For this review, take the finished solid that the model builds, in its own axes (mm). A direction names the side the tool comes from. Round coordinates to 2 decimals unless told otherwise and drop trailing zeros. Order: outer loops, then holes, each group sorted by start corner. A loop starts at its lowest first (then second) coordinate and runs counter-clockwise, first axis right, second up. Notation, with made-up numbers: (-22, 5) -> (17, 5) arc R10 ccw to (17, 22) -> close; hole circle Ø10 at (60, 80.5). An arc over 180 degrees is marked (long way). Put each result on its own line as item: value. Start each with the question number.
```python
from build123d import *

# Parameters (mm, degrees)
F0_W     = 67.1
F0_H     = 138.3
F1_DEPTH = 3.55
F2_R     = 5
F3_T     = -2.5
F4_R     = 5
F6_DEPTH = 25


with BuildPart() as f1:
    # F0 (on Front) → F1 (new body, symmetric)
    with BuildSketch(Plane.XZ):
        with Locations((0, -4.651891)):
            Rectangle(F0_W, F0_H)
    extrude(amount=F1_DEPTH, both=True)

    # F2
    f2_edges = [f1.edges().sort_by_distance(p)[0] for p in [
        (-33.55, 0, 64.498109),
        (33.55, 0, 64.498109),
        (33.55, 0, -73.801891),
        (-33.55, 0, -73.801891),
    ]]
    fillet(f2_edges, radius=F2_R)

    # F3
    f3_openings = [f1.faces().sort_by_distance(p)[0] for p in [
        (0, -3.55, -4.651891),
    ]]
    offset(amount=F3_T, openings=f3_openings)

    # F4
    f4_edges = [f1.edges().sort_by_distance(p)[0] for p in [
        (33.55, 3.55, -4.651891),
        (32.085534, 3.55, -72.337424),
        (32.085534, 3.55, 63.033643),
        (0, 3.55, -73.801891),
        (0, 3.55, 64.498109),
        (-32.085534, 3.55, -72.337424),
        (-32.085534, 3.55, 63.033643),
        (-33.55, 3.55, -4.651891),
    ]]
    fillet(f4_edges, radius=F4_R)

    # F5 (on Front) → F6 (cut)
    with BuildSketch(Plane.XZ):
        with BuildLine():
            add(Edge.make_bspline(
                [(27.755955, 53.217217), (27.755955, 64.267715), (15.384319, 58.742466), (3.012683, 53.217217), (15.384319, 47.691968), (27.755955, 42.166719), (27.755955, 53.217217)],
                knots=[0, 0, 0, 2.094395, 2.094395, 4.18879, 4.18879, 6.283185, 6.283185, 6.283185], degree=2, weights=[1, 0.5, 1, 0.5, 1, 0.5, 1]))
        make_face()
    extrude(amount=-F6_DEPTH, mode=Mode.SUBTRACT)


solid = f1.part
```
Item 1: Mouldability with a two-part tool opening along Z and no side actions: class faces 3 (the face through (-32.12, -2.51, -72.3)), 4 (the face through (-32.124, -2.485, 62.995)), 5 (the face through (-30.337, -1.218, 61.246)) as +Z half, -Z half, draft (parallel to the pull), parting line (faces both ways), or undercut.
Item 2: Consider section B-B, the plane z = -2.5. Write out the cut boundary in (x, y), plus the area to 3 significant figures.
Item 3: Tool access review of faces 1 (the face through (31.05, -1, -6)), 2 (the face through (32.124, -2.485, 62.995)): name each direction out of +Z, -Z, +X, -X, +Y, -Y from which nothing blocks a thin tool from reaching the whole face with its end or side.
Item 4: For L1, parallel to Z at x = -11.5, y = -2; L2, parallel to X at y = -2.25, z = -56.5, list the stretches that pass through material, from the lowest coordinate up.
Item 5: Consider section A-A, the plane x = -11. Write out the cut boundary in (y, z), plus the area to 3 significant figures.
Item 6: Insertion check: pin 1 Ø2 at (x, y) = (0, 0) entering from -Z; pin 2 Ø1 at (x, z) = (-20.5, -37) entering from -Y; pin 3 Ø1.5 at (x, y) = (17, 1) entering from +Z; pin 4 Ø1.4 at (x, y) = (-13.5, -1) entering from +Z. Each pin has a flat end and moves straight along its axis. Give the tip position at first contact, or say it passes through.
Evaluation:
1. face 3: -Z half
1. face 4: +Z half
1. face 5: undercut
2. outline: (-33.55, -3.55) -> (-31.05, -3.55) -> (-31.05, 1.05) -> (31.05, 1.05) -> (31.05, -3.55) -> (33.55, -3.55) -> (33.55, -1.45) arc R5 ccw to (28.55, 3.55) -> (-28.55, 3.55) arc R5 ccw to (-33.55, -1.45) -> close
2. area: 180 mm^2
3. face 1: -Y
3. face 2: +Z, +X, +Y, -Y
4. L1: z = -73.8 to -71.3, 62 to 64.5
4. L2: x = -33.55 to -31.05, 31.05 to 33.55
5. outline: (-3.55, -73.8) -> (-1.45, -73.8) arc R5 ccw to (3.55, -68.8) -> (3.55, 59.5) arc R5 ccw to (-1.45, 64.5) -> (-3.55, 64.5) -> (-3.55, 62) -> (1.05, 62) -> (1.05, -71.3) -> (-3.55, -71.3) -> close
5. area: 358 mm^2
6. pin 1: stops at z = -73.78
6. pin 2: stops at y = 1.05
6. pin 3: stops at z = 64.2
6. pin 4: stops at z = 64.5
